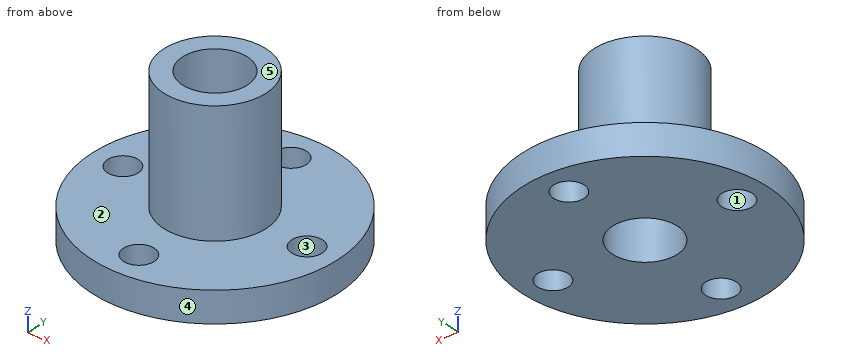
```python
from build123d import *

# Parameters (mm, degrees)
SKETCH1_R           = 12
BOSS_EXTRUDE1_DEPTH = 3
SKETCH2_R           = 5
BOSS_EXTRUDE2_DEPTH = 15
SKETCH3_R           = 3.17
CUT_EXTRUDE1_DEPTH  = 15
SKETCH4_R           = 1.5
CUT_EXTRUDE2_DEPTH  = 5


with BuildPart() as part:
    # Sketch1 → Boss-Extrude1 (new body)
    with BuildSketch(Plane.XY):
        Circle(SKETCH1_R)
    extrude(amount=BOSS_EXTRUDE1_DEPTH)

    # Sketch2 → Boss-Extrude2 (add)
    with BuildSketch(Plane.XY):
        Circle(SKETCH2_R)
    extrude(amount=BOSS_EXTRUDE2_DEPTH)

    # Sketch3 → Cut-Extrude1 (cut)
    with BuildSketch(Plane.XY):
        Circle(SKETCH3_R)
    extrude(amount=CUT_EXTRUDE1_DEPTH, mode=Mode.SUBTRACT)

    # Sketch4 → Cut-Extrude2 (cut)
    with BuildSketch(Plane.XY):
        with Locations((-9, 0)):
            Circle(SKETCH4_R)
        with Locations((0, 9)):
            Circle(SKETCH4_R)
        with Locations((9, 0)):
            Circle(SKETCH4_R)
        with Locations((0, -9)):
            Circle(SKETCH4_R)
    extrude(amount=CUT_EXTRUDE2_DEPTH, mode=Mode.SUBTRACT)


solid = part.part
```
Design review of the part built by this model. Coordinates are the model's own, in mm. Face numbers are marked on the shaded views. A direction names the side the tool comes from. Give positions to 0.01 mm unless a question says otherwise; leave off trailing zeros. Write each loop counter-clockwise with the first axis right and the second up, starting at its lowest first coordinate (ties: lowest second). Pieces come first, ordered by that corner, then holes. Notation, with made-up numbers: (70.5, -21.5) -> (79.5, -21.5) arc R23 cw to (79.5, 6.5) -> close; hole circle Ø11 at (28.25, 64.5). An arc over 180 degrees is marked (long way). Answer in a Markdown table with one row per item.
(1) To check wall thickness, follow probe 1 along Y at (x, z) = (0, 1.65); probe 2 along Y at (x, z) = (0, 11); probe 3 along Z at (x, y) = (4.75, 3.75). State the ranges of each line that lie inside material, in increasing order.
Results:
| item | result |
|---|---|
| probe 1 | -12 to -10.5, -7.5 to -3.17, 3.17 to 7.5, 10.5 to 12 |
| probe 2 | -5 to -3.17, 3.17 to 5 |
| probe 3 | 0 to 3 |
(2) Consider section B-B (x = 2). State the section outline as (y, z) points.
Results:
| item | result |
|---|---|
| outline | (-11.83, 0) -> (-2.46, 0) -> (-2.46, 15) -> (-4.58, 15) -> (-4.58, 3) -> (-11.83, 3) -> close; (2.46, 0) -> (11.83, 0) -> (11.83, 3) -> (4.58, 3) -> (4.58, 15) -> (2.46, 15) -> close |
(3) Clearance check with flat-ended pins moving along their axes: pin 1 (2 mm diameter, centred on y = 4, z = 9.5, fed in from +X); pin 2 (8 mm diameter, centred on x = -8.5, z = 10, fed in from +Y); pin 3 (2.5 mm diameter, centred on x = 0, y = 9, fed in from +Z); pin 4 (5 mm diameter, centred on y = 1, z = 6.5, fed in from +X). State where each tip first meets the part, or that it passes through.
Results:
| item | result |
|---|---|
| pin 1 | x = 4 |
| pin 2 | y = 2.18 |
| pin 3 | through |
| pin 4 | x = 5 |
(4) Consider section A-A (y = 0). State the section outline as (x, z) points, then the cut area to 3 significant figures.
Results:
| item | result |
|---|---|
| outline | (-12, 0) -> (-10.5, 0) -> (-10.5, 3) -> (-12, 3) -> close; (-7.5, 0) -> (-3.17, 0) -> (-3.17, 15) -> (-5, 15) -> (-5, 3) -> (-7.5, 3) -> close; (3.17, 0) -> (7.5, 0) -> (7.5, 3) -> (5, 3) -> (5, 15) -> (3.17, 15) -> close; (10.5, 0) -> (12, 0) -> (12, 3) -> (10.5, 3) -> close |
| area | 78.9 mm2 |
(5) Consider section D-D (x = -3.5). State the section outline as (y, z) points, then the cut area to 3 significant figures.
Results:
| item | result |
|---|---|
| outline | (-11.48, 0) -> (11.48, 0) -> (11.48, 3) -> (3.57, 3) -> (3.57, 15) -> (-3.57, 15) -> (-3.57, 3) -> (-11.48, 3) -> close |
| area | 155 mm2 |
(6) For the marked faces 1 and 2, list the 3-axis set-ups (+Z, -Z, +X, -X, +Y, -Y) from which the entire face can be reached by the end or side of a thin tool; tool diameter is ignored.
Results:
| item | result |
|---|---|
| face 1 | +Z, -Z |
| face 2 | +Z |
(7) Consider section C-C (y = 8.25). State the section outline as (x, z) points, then the cut area to 3 significant figures.
Results:
| item | result |
|---|---|
| outline | (-8.71, 0) -> (-1.3, 0) -> (-1.3, 3) -> (-8.71, 3) -> close; (1.3, 0) -> (8.71, 0) -> (8.71, 3) -> (1.3, 3) -> close |
| area | 44.5 mm2 |
(8) Mouldability with a two-part tool opening along Y and no side actions: class the marked faces 3, 4 and 5 as +Y half, -Y half, draft (parallel to the pull), parting line (faces both ways), or undercut.
Results:
| item | result |
|---|---|
| face 3 | undercut |
| face 4 | parting line |
| face 5 | draft |
